Build history of the part. All positions in model axes, mm. A direction names the side the tool comes from. Give positions to 0.01 mm unless a question says otherwise; leave off trailing zeros. Order: outer loops, then holes, each group sorted by start corner. A loop starts at its lowest first (then second) coordinate and runs counter-clockwise, first axis right, second up. Notation, with made-up numbers: (71, 56.25) - (112, 56.25) arc R19 cw to (112, 87.25) - close; hole circle Ø10 at (27, 53.25). An arc over 180 degrees is marked (long way). One line per item, written item: value.
```python
from build123d import *

# Parameters (mm, degrees)
SKETCH_1_W          = 71
SKETCH_1_H          = 93
SKETCH_1_R          = 1.6
SKETCH_1_W_2        = 51
SKETCH_1_H_2        = 78.2
EXTRUDE_1_DEPTH     = 5
SKETCH_2_W          = 71
SKETCH_2_H          = 93
SKETCH_2_W_2        = 70.5
SKETCH_2_H_2        = 92.5
CUT_EXTRUDE_1_DEPTH = 6
SKETCH_3_W          = 51.5
SKETCH_3_H          = 78.7
SKETCH_3_W_2        = 51
SKETCH_3_H_2        = 78.2
CUT_EXTRUDE_2_DEPTH = 6
SKETCH_5_W          = 27
SKETCH_5_H          = 92.5
SKETCH_5_R          = 1.6
EXTRUDE_3_DEPTH     = 2


with BuildPart() as part:
    # Эскиз1 → Бобышка-Вытянуть1 (new body)
    with BuildSketch(Plane(origin=(0, 0, 28), x_dir=(-1, 0, 0), z_dir=(0, 0, -1))):
        with Locations((-39.5, 51)):
            Rectangle(SKETCH_1_W, SKETCH_1_H)
        with Locations((-6.6, 7.5)):
            Circle(SKETCH_1_R, mode=Mode.SUBTRACT)
        with Locations((-72.4, 7.5)):
            Circle(SKETCH_1_R, mode=Mode.SUBTRACT)
        with Locations((-6.6, 94.5)):
            Circle(SKETCH_1_R, mode=Mode.SUBTRACT)
        with Locations((-72.4, 94.5)):
            Circle(SKETCH_1_R, mode=Mode.SUBTRACT)
        with Locations((-38.9, 51)):
            Rectangle(SKETCH_1_W_2, SKETCH_1_H_2, mode=Mode.SUBTRACT)
    extrude(amount=EXTRUDE_1_DEPTH)

    # Эскиз2 → Вырез-Вытянуть1 (cut, through all)
    with BuildSketch(Plane.XY.offset(28)):
        with Locations((39.5, 51)):
            Rectangle(SKETCH_2_W, SKETCH_2_H)
        with Locations((39.5, 51)):
            Rectangle(SKETCH_2_W_2, SKETCH_2_H_2, mode=Mode.SUBTRACT)
    extrude(amount=-CUT_EXTRUDE_1_DEPTH, mode=Mode.SUBTRACT)

    # Эскиз3 → Вырез-Вытянуть2 (cut, through all)
    with BuildSketch(Plane.XY.offset(28)):
        with Locations((38.9, 51)):
            Rectangle(SKETCH_3_W, SKETCH_3_H)
        with Locations((38.9, 51)):
            Rectangle(SKETCH_3_W_2, SKETCH_3_H_2, mode=Mode.SUBTRACT)
    extrude(amount=-CUT_EXTRUDE_2_DEPTH, mode=Mode.SUBTRACT)

    # Эскиз5 → Бобышка-Вытянуть3 (add)
    with BuildSketch(Plane(origin=(0, 0, 23), x_dir=(-1, 0, 0), z_dir=(0, 0, -1))):
        with Locations((-78.15, 51)):
            Rectangle(SKETCH_5_W, SKETCH_5_H)
        with Locations((-72.4, 94.5)):
            Circle(SKETCH_5_R, mode=Mode.SUBTRACT)
        with Locations((-72.4, 7.5)):
            Circle(SKETCH_5_R, mode=Mode.SUBTRACT)
    extrude(amount=EXTRUDE_3_DEPTH)


solid = part.part
```
(1) 3-axis set-ups, long thin cutter, end or side, ignore diameter. For faces 4 (the face through (74.75, 50, 26)), 5 (the face through (13.15, 50, 26)), 6 (the face through (12, 48, 23)): which of +Z, -Z, +X, -X, +Y, -Y reach the whole face in a straight line?
Completed:
face 4: +Z, +X, +Y, -Y
face 5: +Z, -Z
face 6: -Z, -X, +Y, -Y
(2) Slice it at B-B, the plane y = 19. Give the cut face in (x, z), and give its area (3 significant figures).
Completed:
outline: (4.25, 23) - (13.15, 23) - (13.15, 28) - (4.25, 28) - close; (64.65, 21) - (91.65, 21) - (91.65, 23) - (74.75, 23) - (74.75, 28) - (64.65, 28) - close
area: 149 mm²
(3) Slice it at C-C, the plane x = 6.6. Give the cut face in (y, z).
Completed:
outline: (4.75, 23) - (5.9, 23) - (5.9, 28) - (4.75, 28) - close; (9.1, 23) - (92.9, 23) - (92.9, 28) - (9.1, 28) - close; (96.1, 23) - (97.25, 23) - (97.25, 28) - (96.1, 28) - close
(4) Slice it at A-A, the plane x = 62. Give the cut face in (y, z), and give its area (3 significant figures).
Completed:
outline: (4.75, 23) - (11.65, 23) - (11.65, 28) - (4.75, 28) - close; (90.35, 23) - (97.25, 23) - (97.25, 28) - (90.35, 28) - close
area: 69.0 mm²
(5) Pin check, flat tips, straight feed: P1, Ø12, axis at x = 57.5, y = 26, coming from the +Z side; P2, Ø5, axis at x = 80.5, y = 47, coming from the +Z side; P3, Ø1.5, axis at y = 69, z = 25, coming from the +X side; P4, Ø5, axis at x = 6.6, y = 94.5, coming from the -Z side. Stop position of each tip, or through.
Completed:
P1: through
P2: z = 23
P3: x = 74.75
P4: z = 23
(6) Pull direction X, two halves, no side cores. Call faces 1 (the face through (6.808, 96.086, 25.535)), 2 (the face through (4.25, 50, 26)), 3 (the face through (83, 52, 23)): +X half, -X half, draft (parallel to the pull), parting line (faces both ways), or undercut.
Completed:
face 1: undercut
face 2: -X half
face 3: draft
(7) Drill centre lines: line 1 (X direction, y = 94.5, z = 25.25); line 2 (Y direction, x = 6.6, z = 24.95); line 3 (Y direction, x = 38, z = 27.25). Where is each one in solid material? Low to high.
Completed:
line 1: 4.25 to 5, 8.2 to 70.8, 74 to 74.75
line 2: 4.75 to 5.9, 9.1 to 92.9, 96.1 to 97.25
line 3: 4.75 to 11.65, 90.35 to 97.25
(8) Slice it at D-D, the plane z = 24.5. Give the cut face in (x, y).
Completed:
outline: (4.25, 4.75) - (74.75, 4.75) - (74.75, 97.25) - (4.25, 97.25) - close; hole circle Ø3.2 at (6.6, 7.5); hole circle Ø3.2 at (6.6, 94.5); hole (13.15, 11.65) - (64.65, 11.65) - (64.65, 90.35) - (13.15, 90.35) - close; hole circle Ø3.2 at (72.4, 7.5); hole circle Ø3.2 at (72.4, 94.5)
